```python
from build123d import *

# Parameters (mm, degrees)
F5_ANGLE_BACK = 10
F5_ANGLE      = 20
F3_DEPTH      = 15
F1_R          = 5
F4_DEPTH      = 61.9


with BuildPart() as f5:
    # F0 (on Front) → F5 (revolve)
    with BuildSketch(Plane.XZ, mode=Mode.PRIVATE) as f5_sk:
        Polygon((69.7967915205, 0), (60.5548890955, 15), (54.7967915205, 15), (54.7967915205, 0), align=None)
    revolve(f5_sk.sketch.rotate(Axis((0, 0, 12.625), (0, 0, 1)), -F5_ANGLE_BACK), axis=Axis((0, 0, 12.625), (0, 0, 1)), revolution_arc=F5_ANGLE)

    # F2 (on face) → F3 (join)
    with BuildSketch(Plane.XY.offset(15)):
        Polygon((54.7967915205, 9.6621528013), (53.9643051295, 9.5153629895), (53.9643051295, -9.5153629895), (54.7967915205, -9.6621528013), (56.5004897511, 0), align=None)
    extrude(amount=-F3_DEPTH)

    # F1 (on Right) → F4 (cut)
    with BuildSketch(Plane.YZ):
        with Locations((0, 7.5)):
            Circle(F1_R)
    extrude(amount=F4_DEPTH, mode=Mode.SUBTRACT)


solid = f5.part
```
Read the model definition and answer for the solid it produces. Units are mm, in the model's axes. A direction names the side the tool comes from. Coordinates: 2 decimals unless noted, no trailing zeros. Order: outer loops, then holes, each group sorted by start corner. A loop starts at its lowest first (then second) coordinate and runs counter-clockwise, first axis right, second up. Notation, with made-up numbers: (7.5, 19) - (62.5, 19) arc R19 ccw to (62.5, 36) - close; hole circle Ø1 at (26.5, 71.5). An arc over 180 degrees is marked (long way). Answer as a JSON object with one key per item and string values. Group by question number.
Item 1: The mould has two halves that part along Y. Classify faces 3 (the face through (61.9, 0, 8)), 4 (the face through (57, 1, 15)), 5 (the face through (65.111, -0.159, 7.605)): +Y half, -Y half, draft (parallel to the pull), parting line (faces both ways), or undercut.
Item 2: Section A-A (y = 0) is taken. Give the vertices of the cut face in (x, z).
Item 3: Flat-ended cylindrical pins translate along their axes: P1, Ø2, axis at y = -7, z = 9, coming from the +X side; P2, Ø3, axis at y = 1, z = 9.5, coming from the -X side; P3, Ø1, axis at y = 9, z = 3.5, coming from the +X side. Find the tip coordinate at first contact, or state that the pin passes through.
Item 4: A tool of negligible diameter and unlimited length cuts with its end or side. For faces 1 (the face through (53.964, 0, 13)), 2 (the face through (57.877, -0.651, 12.457)), from which of +Z, -Z, +X, -X, +Y, -Y can it reach the whole face along a straight path? Write none if from no direction.
Item 5: Section C-C (z = 8.25) is taken. Give the vertices of the cut face in (x, y).
Item 6: Section B-B (x = 58.25) is taken. Give the vertices of the cut face in (y, z), plus the area to 3 significant figures.
Item 7: Section D-D (x = 56.5) is taken. Give the vertices of the cut face in (y, z), plus the area to 3 significant figures.
Item 8: Consider probe 1 along Z at (x, y) = (60, 0); probe 2 along Y at (x, z) = (55.5, 7.5); probe 3 along Y at (x, z) = (56.5, 7.5). Determine where each line is inside the solid, lowest interval first. Write a range as from..to.
Results are:
{
 "1": {"face 3": "undercut", "face 4": "draft", "face 5": "parting line"},
 "2": {"outline": "(53.96, 0) - (69.8, 0) - (60.55, 15) - (53.96, 15) - (53.96, 12.5) - (61.9, 12.5) - (61.9, 2.5) - (53.96, 2.5) - close"},
 "3": {"P1": "stops at x = 64.5", "P2": "stops at x = 61.9", "P3": "stops at x = 67.36"},
 "4": {"face 1": "+Z, -Z, -X, +Y, -Y", "face 2": "-X"},
 "5": {"outline": "(53.96, -9.52) - (63.73, -11.24) arc R64.71 ccw to (63.73, 11.24) - (53.96, 9.52) - (53.96, 4.94) - (61.9, 4.94) - (61.9, -4.94) - (53.96, -4.94) - close"},
 "6": {"outline": "(-10.27, 0) - (10.27, 0) - (10.27, 15) - (-10.27, 15) - close; hole circle Ø10 at (0, 7.5)", "area": "230 mm^2"},
 "7": {"outline": "(-9.96, 0) - (9.96, 0) - (9.96, 15) - (-9.96, 15) - close; hole circle Ø10 at (0, 7.5)", "area": "220 mm^2"},
 "8": {"probe 1": "z = 0..2.5, 12.5..15", "probe 2": "y = -9.79..-5, 5..9.79", "probe 3": "y = -9.96..-5, 5..9.96"}
}
